from build123d import *

# Parameters (mm, degrees)
BOSS_EXTRUDE1_DEPTH = 100
FILLET1_R           = 1
SKETCH2_R           = 2
CUT_EXTRUDE1_DEPTH  = 10


with BuildPart() as part:
    # Sketch1 → Boss-Extrude1 (new body)
    with BuildSketch(Plane(origin=(0, 0, 0), x_dir=(1, 0, 0), z_dir=(0, 1, 0))):
        Polygon((0, 0), (15, 0), (15, -2), (15, -10), (7, -10), (0, -10), (0, -7), (5, -7), (5, -2), (0, -2), align=None)
    extrude(amount=BOSS_EXTRUDE1_DEPTH)

    # Fillet1
    fillet1_edges = [part.edges().sort_by_distance(p)[0] for p in [
        (15, 50, 10),
        (0, 50, 7),
        (0, 50, 2),
    ]]
    fillet(fillet1_edges, radius=FILLET1_R)

    # Sketch2 → Cut-Extrude1 (cut)
    with BuildSketch(Plane.XY.offset(10)):
        with Locations((10, 16.7)):
            Circle(SKETCH2_R)
        with Locations((10, 83.3)):
            Circle(SKETCH2_R)
        with Locations((10, 50)):
            Circle(SKETCH2_R)
    extrude(amount=-CUT_EXTRUDE1_DEPTH, mode=Mode.SUBTRACT)


solid = part.part
Can you work these out from the model? Positions are in its coordinate system, mm. A direction names the side the tool comes from. Round coordinates to 2 decimals unless told otherwise and drop trailing zeros. Order: outer loops, then holes, each group sorted by start corner. A loop starts at its lowest first (then second) coordinate and runs counter-clockwise, first axis right, second up. Notation, with made-up numbers: (13.25, -12.75) -> (40.25, -12.75) arc R10 ccw to (40.25, 4.25) -> close; hole circle Ø1 at (-8.75, -12). An arc over 180 degrees is marked (long way). Write each question's results on one line, items separated by ' | '. Start each with the question number.
Item 1: If we section it at C-C, the plane z = 4.25: Write out the boundary of the cut face in (x, y).
Item 2: Thinking about a two-plate mould opening in X: for faces 1 (the flat face through (9, 100, 5)), 2 (the cylindrical face through (9.566, 14.748, 5.07)), 3 (the flat face through (15, 49, 5)), 4 (the cylindrical face through (10.923, 48.226, 5.07)), which applies, +X half, -X half, draft (parallel to the pull), parting line (faces both ways), or undercut?
Item 3: Will these pins go through, and if not, where does the flat tip stop? pin 1 (8 mm diameter, centred on x = 6, y = 38.5, fed in from -Z); pin 2 (1.5 mm diameter, centred on y = 47.5, z = 5.5, fed in from -X).
Item 4: Please list where these lines run through material, in increasing order: L1, parallel to Y at x = 10, z = 3.5; L2, parallel to Z at x = 4.75, y = 25.5; L3, parallel to X at y = 89, z = 5.5.
Item 5: If we section it at B-B, the plane x = 10: Write out the boundary of the cut face in (y, z), then the cut area to 3 significant figures.
Item 6: If we section it at A-A, the plane y = 83.3: Write out the boundary of the cut face in (x, z).
Item 7: If we section it at D-D, the plane y = 34.5: Write out the boundary of the cut face in (x, z).
Item 8: Which directions (+Z, -Z, +X, -X, +Y, -Y) give clear straight access to the entire face, cutting with the end or side of a thin tool? Please do faces 5 (the flat face through (0, 49, 9)), 6 (the flat face through (3, 49, 7)).
Results:
1) outline: (5, 0) -> (15, 0) -> (15, 100) -> (5, 100) -> close; hole circle Ø4 at (10, 16.7); hole circle Ø4 at (10, 50); hole circle Ø4 at (10, 83.3)
2) face 1: draft | face 2: undercut | face 3: +X half | face 4: undercut
3) pin 1: stops at z = 0 | pin 2: stops at x = 5
4) L1: y = 0 to 14.7, 18.7 to 48, 52 to 81.3, 85.3 to 100 | L2: z = 0 to 2, 7 to 10 | L3: x = 5 to 15
5) outline: (0, 0) -> (14.7, 0) -> (14.7, 10) -> (0, 10) -> close; (18.7, 0) -> (48, 0) -> (48, 10) -> (18.7, 10) -> close; (52, 0) -> (81.3, 0) -> (81.3, 10) -> (52, 10) -> close; (85.3, 0) -> (100, 0) -> (100, 10) -> (85.3, 10) -> close | area: 880 mm2
6) outline: (0, 0) -> (8, 0) -> (8, 10) -> (0, 10) -> (0, 8) arc R1 ccw to (1, 7) -> (5, 7) -> (5, 2) -> (1, 2) arc R1 ccw to (0, 1) -> close; (12, 0) -> (15, 0) -> (15, 9) arc R1 ccw to (14, 10) -> (12, 10) -> close
7) outline: (0, 0) -> (15, 0) -> (15, 9) arc R1 ccw to (14, 10) -> (0, 10) -> (0, 8) arc R1 ccw to (1, 7) -> (5, 7) -> (5, 2) -> (1, 2) arc R1 ccw to (0, 1) -> close
8) face 5: +Z, -Z, -X, +Y, -Y | face 6: -X, +Y, -Y
